from build123d import *

# Parameters (mm, degrees)
SKETCH1_R              = 20
BOSS_EXTRUDE2_DEPTH    = 8
SKETCH7_R              = 20
BOSS_EXTRUDE3_DEPTH    = 5
CUT_EXTRUDE2_START     = -20.000000091
CUT_EXTRUDE2_OUTLINE_R = 2
CUT_EXTRUDE2_DEPTH     = 20.00000009
SKETCH14_R             = 1.5
CUT_EXTRUDE3_DEPTH     = 25
SKETCH15_R             = 17
CUT_EXTRUDE4_DEPTH     = 10


# Read off the part's stored shape, not the designer's step: Cut-Extrude2
with BuildPart() as part:
    # Sketch1 → Boss-Extrude2 (new body)
    with BuildSketch(Plane(origin=(0, 0, 0), x_dir=(1, 0, 0), z_dir=(0, 1, 0))):
        with Locations(Location((0, 0, 0), (0, 0, 270))):
            Circle(SKETCH1_R)
    extrude(amount=BOSS_EXTRUDE2_DEPTH)

    # Sketch7 → Boss-Extrude3 (add)
    with BuildSketch(Plane(origin=(0, 8, 0), x_dir=(1, 0, 0), z_dir=(0, 1, 0))):
        with Locations(Location((0, 0, 0), (0, 0, 270))):
            Circle(SKETCH7_R)
    extrude(amount=BOSS_EXTRUDE3_DEPTH)

    # Cut-Extrude2 outline → Cut-Extrude2 (cut)
    with BuildSketch(Plane(origin=(0, 0, 0), x_dir=(0.5840722771163888, 0, 0.8117016539986083), z_dir=(0.8117016539986082, 0, -0.5840722771163891)).offset(CUT_EXTRUDE2_START)):
        with Locations((0, -8)):
            Circle(CUT_EXTRUDE2_OUTLINE_R)
    extrude(amount=CUT_EXTRUDE2_DEPTH, mode=Mode.SUBTRACT)

    # Sketch14 → Cut-Extrude3 (cut)
    with BuildSketch(Plane(origin=(0, 0, 0), x_dir=(0.5840722775801191, 0, 0.8117016536649241), z_dir=(-0.8117016536649241, 0, 0.5840722775801191))):
        with Locations((0, 8)):
            Circle(SKETCH14_R)
    extrude(amount=-CUT_EXTRUDE3_DEPTH, mode=Mode.SUBTRACT)

    # Sketch15 → Cut-Extrude4 (cut)
    with BuildSketch(Plane(origin=(0, 13, 0), x_dir=(1, 0, 0), z_dir=(0, 1, 0))):
        with Locations(Location((0, 0, 0), (0, 0, 270))):
            Circle(SKETCH15_R)
    extrude(amount=-CUT_EXTRUDE4_DEPTH, mode=Mode.SUBTRACT)


solid = part.part
Design review of the part built by this model. Coordinates are the model's own, in mm. A direction names the side the tool comes from. Coordinates: 2 decimals unless noted, no trailing zeros. Order: outer loops, then holes, each group sorted by start corner. A loop starts at its lowest first (then second) coordinate and runs counter-clockwise, first axis right, second up. Notation, with made-up numbers: (56.25, -5) -> (70.25, -5) arc R32 cw to (70.25, 24) -> close; hole circle Ø10 at (19, 11.25). An arc over 180 degrees is marked (long way). One line per item, written item: value.
1) Clearance check with flat-ended pins moving along their axes: P1, Ø1.5, axis at y = 3.5, z = 6, coming from the -X side; P2, Ø5, axis at y = 2.5, z = -12.5, coming from the -X side; P3, Ø1, axis at y = 8.5, z = 14.5, coming from the +X side. State where each tip first meets the part, or that it passes through.
Output values:
P1: stops at x = -19.3
P2: stops at x = -17.32
P3: stops at x = 14.28
2) Draft analysis for pull direction X (two halves, no side actions). For faces 3 (the face through (0, 0, 0)), 4 (the face through (-19.524, 6.409, -4.336)), 5 (the face through (0, 3, 0)), state which applies: +X half, -X half, draft (parallel to the pull), parting line (faces both ways), or undercut.
Output values:
face 3: draft
face 4: parting line
face 5: undercut
3) We need section A-A, the plane x = 0. Give the boundary of the cut face in (y, z).
Output values:
outline: (0, -20) -> (13, -20) -> (13, -17) -> (3, -17) -> (3, 17) -> (13, 17) -> (13, 20) -> (0, 20) -> close
4) Machinability: for faces 1 (the face through (16.855, 8.07, -2.213)), 2 (the face through (-15, 13, -9)), which of the approach directions +Z, -Z, +X, -X, +Y, -Y give a long, thin tool a straight path to every point of the face, cutting with its end or side? Answer none if there is none.
Output values:
face 1: +Y
face 2: +Z, -Z, +X, -X, +Y
5) We need section B-B, the plane z = 0. Give the boundary of the cut face in (x, y), then the cut area to 3 significant figures.
Output values:
outline: (-20, 0) -> (20, 0) -> (20, 13) -> (17, 13) -> (17, 3) -> (-17, 3) -> (-17, 13) -> (-20, 13) -> close
area: 180 mm2
6) We need section C-C, the plane y = 1. Give the boundary of the cut face in (x, z), then the cut area to 3 significant figures.
Output values:
outline: circle Ø40 at (0, 0)
area: 1,260 mm2
7) To check wall thickness, follow probe 1 along Y at (x, z) = (-5.5, -3); probe 2 along X at (y, z) = (8.25, 0); probe 3 along Z at (x, y) = (11, 3.5). State the ranges of each line that lie inside material, in increasing order. Write a range as [from, to].
Output values:
probe 1: y = [0, 3]
probe 2: x = [-20, -17], [17, 20]
probe 3: z = [-16.7, -12.96], [12.96, 16.7]
